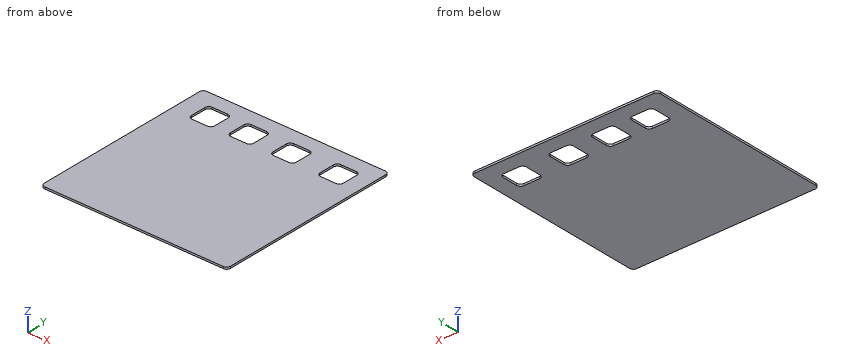
```python
from build123d import *

# Parameters (mm, degrees)
F1_DEPTH = 3.175
F3_DEPTH = 3.175


with BuildPart() as f1:
    # F0 (on Top) → F1 (new body)
    with BuildSketch(Plane.XY):
        with BuildLine():
            ThreePointArc((152.4, 146.05), (150.540128, 150.540128), (146.05, 152.4))
            Line((146.05, 152.4), (-146.05, 152.4))
            ThreePointArc((-146.05, 152.4), (-150.540128, 150.540128), (-152.4, 146.05))
            Line((-152.4, 146.05), (-152.4, -146.05))
            ThreePointArc((-152.4, -146.05), (-150.540128, -150.540128), (-146.05, -152.4))
            Line((-146.05, -152.4), (146.05, -152.4))
            ThreePointArc((146.05, -152.4), (150.540128, -150.540128), (152.4, -146.05))
            Line((152.4, -146.05), (152.4, 146.05))
        make_face()
    extrude(amount=F1_DEPTH)

    # F2 (on face) → F3 (cut, through all)
    with BuildSketch(Plane.XY.offset(3.175)):
        with BuildLine():
            Line((-115.838222, 89.799137), (-90.438222, 89.799137))
            ThreePointArc((-90.438222, 89.799137), (-85.948094, 91.659008), (-84.088222, 96.149137))
            Line((-84.088222, 96.149137), (-84.088222, 121.549137))
            ThreePointArc((-84.088222, 121.549137), (-85.948094, 126.039265), (-90.438222, 127.899137))
            Line((-90.438222, 127.899137), (-115.838222, 127.899137))
            ThreePointArc((-115.838222, 127.899137), (-120.32835, 126.039265), (-122.188222, 121.549137))
            Line((-122.188222, 121.549137), (-122.188222, 96.149137))
            ThreePointArc((-122.188222, 96.149137), (-120.32835, 91.659008), (-115.838222, 89.799137))
        make_face()
        with BuildLine():
            Line((-52.185156, 89.799137), (-26.785156, 89.799137))
            ThreePointArc((-26.785156, 89.799137), (-22.295028, 91.659008), (-20.435156, 96.149137))
            Line((-20.435156, 96.149137), (-20.435156, 121.549137))
            ThreePointArc((-20.435156, 121.549137), (-22.295028, 126.039265), (-26.785156, 127.899137))
            Line((-26.785156, 127.899137), (-52.185156, 127.899137))
            ThreePointArc((-52.185156, 127.899137), (-56.675284, 126.039265), (-58.535156, 121.549137))
            Line((-58.535156, 121.549137), (-58.535156, 96.149137))
            ThreePointArc((-58.535156, 96.149137), (-56.675284, 91.659008), (-52.185156, 89.799137))
        make_face()
        with BuildLine():
            Line((94.603679, 89.799137), (120.003679, 89.799137))
            ThreePointArc((120.003679, 89.799137), (124.493807, 91.659008), (126.353679, 96.149137))
            Line((126.353679, 96.149137), (126.353679, 121.549137))
            ThreePointArc((126.353679, 121.549137), (124.493807, 126.039265), (120.003679, 127.899137))
            Line((120.003679, 127.899137), (94.603679, 127.899137))
            ThreePointArc((94.603679, 127.899137), (90.113551, 126.039265), (88.253679, 121.549137))
            Line((88.253679, 121.549137), (88.253679, 96.149137))
            ThreePointArc((88.253679, 96.149137), (90.113551, 91.659008), (94.603679, 89.799137))
        make_face()
        with BuildLine():
            Line((17.579446, 89.799137), (42.979446, 89.799137))
            ThreePointArc((42.979446, 89.799137), (47.469574, 91.659008), (49.329446, 96.149137))
            Line((49.329446, 96.149137), (49.329446, 121.549137))
            ThreePointArc((49.329446, 121.549137), (47.469574, 126.039265), (42.979446, 127.899137))
            Line((42.979446, 127.899137), (17.579446, 127.899137))
            ThreePointArc((17.579446, 127.899137), (13.089318, 126.039265), (11.229446, 121.549137))
            Line((11.229446, 121.549137), (11.229446, 96.149137))
            ThreePointArc((11.229446, 96.149137), (13.089318, 91.659008), (17.579446, 89.799137))
        make_face()
    extrude(amount=-F3_DEPTH, mode=Mode.SUBTRACT)


solid = f1.part
```
Model file for the job. Use its own axes, mm. Coordinates: 2 decimals unless noted, no trailing zeros. Write each loop counter-clockwise with the first axis right and the second up, starting at its lowest first coordinate (ties: lowest second). Pieces come first, ordered by that corner, then holes. Notation, with made-up numbers: (12.5, 13.5) - (69.5, 13.5) arc R25 cw to (69.5, 45.5) - close; hole circle Ø6 at (66.5, 19). An arc over 180 degrees is marked (long way). Use a Markdown table: item, result. Add a question column.
Item 1: Band-saw the part on B-B, the plane z = 0.95. Give the number of separate pieces and of enclosed holes in the cut face, and give its area (3 significant figures).
Item 2: Band-saw the part on A-A, the plane x = -45. Write the cut outline in (y, z) (3 decimals), and give its area (3 significant figures).
Item 3: Drill centre lines: line 1 along Y through (x, z) = (-51, 2.45); line 2 along Y through (x, z) = (-85.5, 1.95). Where is each one in solid material? Low to high.
A:
| question | item | result |
|---|---|---|
| 1 | separate pieces | 1 |
| 1 | enclosed holes | 4 |
| 1 | area | 87,200 mm² |
| 2 | outline | (-152.4, 0) - (89.799, 0) - (89.799, 3.175) - (-152.4, 3.175) - close; (127.899, 0) - (152.4, 0) - (152.4, 3.175) - (127.899, 3.175) - close |
| 2 | area | 847 mm² |
| 3 | line 1 | y = -152.4 to 89.8, 127.9 to 152.4 |
| 3 | line 2 | y = -152.4 to 92.16, 125.54 to 152.4 |
